Verification items for the finished model (mm, model axes). Face numbers are marked on the shaded views. Give positions to 0.01 mm unless a question says otherwise; leave off trailing zeros. Loops run counter-clockwise (first coordinate to the right, second up) from the corner with the lowest first, then second, coordinate; pieces in that order, holes last. Notation, with made-up numbers: (-0.75, -19) - (8.25, -19) arc R11 cw to (8.25, -1) - close; hole circle Ø2 at (83, 21). An arc over 180 degrees is marked (long way). Answer in a Markdown table with one row per item.
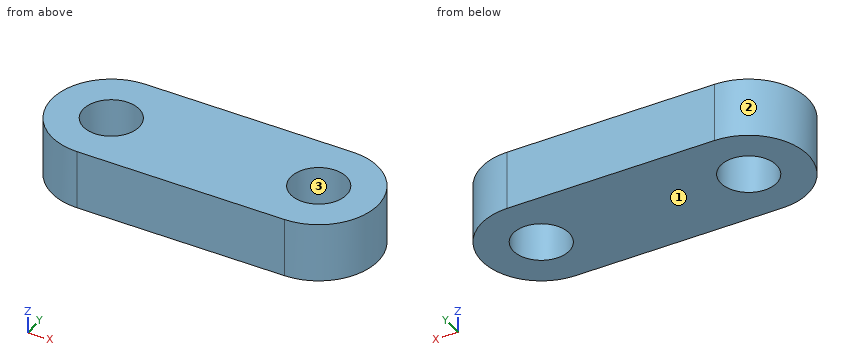
```python
from build123d import *

# Parameters (mm, degrees)
F0_R     = 11.938
F1_DEPTH = 25.4


with BuildPart() as f1:
    # F0 (on Top) → F1 (new body)
    with BuildSketch(Plane.XY):
        with BuildLine():
            Line((44.45, 25.4), (-44.45, 25.4))
            ThreePointArc((-44.45, 25.4), (-69.85, 0), (-44.45, -25.4))
            Line((-44.45, -25.4), (44.45, -25.4))
            ThreePointArc((44.45, -25.4), (69.85, 0), (44.45, 25.4))
        make_face()
        with Locations((-44.45, 0)):
            Circle(F0_R, mode=Mode.SUBTRACT)
        with Locations((44.45, 0)):
            Circle(F0_R, mode=Mode.SUBTRACT)
    extrude(amount=-F1_DEPTH)


solid = f1.part
```
Q1. Thickness scan on line 1 (Y direction, x = 44.45, z = -7.25); line 2 (X direction, y = 6.5, z = -21.5); line 3 (X direction, y = -11, z = -10.5). Record the ranges inside material, lowest first.
Completed:
| item | result |
|---|---|
| line 1 | -25.4 to -11.94, 11.94 to 25.4 |
| line 2 | -69 to -54.46, -34.44 to 34.44, 54.46 to 69 |
| line 3 | -67.34 to -49.09, -39.81 to 39.81, 49.09 to 67.34 |
Q2. Go/stop test with flat-tipped pins: P1, Ø3, axis at y = 4, z = -9, coming from the +X side; P2, Ø10, axis at y = 2.5, z = -6, coming from the -X side; P3, Ø4, axis at y = 9.5, z = -8, coming from the +X side; P4, Ø21.5, axis at x = -44.45, y = 0, coming from the +Z side. Record where each tip stops, or that it passes through.
Completed:
| item | result |
|---|---|
| P1 | x = 69.73 |
| P2 | x = -69.85 |
| P3 | x = 68.72 |
| P4 | through |
Q3. Sectioned sample at C-C (z = -21). Record the cut outline in (x, y), and give its area (3 significant figures).
Completed:
| item | result |
|---|---|
| outline | (-44.45, -25.4) - (44.45, -25.4) arc R25.4 ccw to (44.45, 25.4) - (-44.45, 25.4) arc R25.4 ccw to start; hole circle Ø23.88 at (-44.45, 0); hole circle Ø23.88 at (44.45, 0) |
| area | 5,650 mm^2 |
Q4. Sectioned sample at B-B (x = 38.5). Record the cut outline in (y, z), and give its area (3 significant figures).
Completed:
| item | result |
|---|---|
| outline | (-25.4, -25.4) - (-10.35, -25.4) - (-10.35, 0) - (-25.4, 0) - close; (10.35, -25.4) - (25.4, -25.4) - (25.4, 0) - (10.35, 0) - close |
| area | 765 mm^2 |
Q5. Sectioned sample at D-D (y = -7). Record the cut outline in (x, z), and give its area (3 significant figures).
Completed:
| item | result |
|---|---|
| outline | (-68.87, -25.4) - (-54.12, -25.4) - (-54.12, 0) - (-68.87, 0) - close; (-34.78, -25.4) - (34.78, -25.4) - (34.78, 0) - (-34.78, 0) - close; (54.12, -25.4) - (68.87, -25.4) - (68.87, 0) - (54.12, 0) - close |
| area | 2,520 mm^2 |
Q6. Sectioned sample at A-A (y = 0). Record the cut outline in (x, z), and give its area (3 significant figures).
Completed:
| item | result |
|---|---|
| outline | (-69.85, -25.4) - (-56.39, -25.4) - (-56.39, 0) - (-69.85, 0) - close; (-32.51, -25.4) - (32.51, -25.4) - (32.51, 0) - (-32.51, 0) - close; (56.39, -25.4) - (69.85, -25.4) - (69.85, 0) - (56.39, 0) - close |
| area | 2,340 mm^2 |
Q7. Draft check along Y on the marked faces 1, 2 and 3. Enter one of: +Y half, -Y half, draft (parallel to the pull), parting line (faces both ways), or undercut.
Completed:
| item | result |
|---|---|
| face 1 | draft |
| face 2 | parting line |
| face 3 | undercut |
